```python
from build123d import *

# Parameters (mm, degrees)
SKETCH1_R           = 0.59563
SKETCH1_R_2         = 0.80645
BOSS_EXTRUDE1_DEPTH = 1.5
FILLET2_R           = 22
FILLET3_R           = 28
FILLET1_R           = 1


with BuildPart() as part:
    # Sketch1 → Boss-Extrude1 (new body)
    with BuildSketch(Plane.XY):
        Polygon((-2.5, -3.125), (-2.5, 3.875), (-2.5, 32.875), (27.5, 32.875), (27.5, 46.875), (32.5, 46.875), (32.5, 32.875), (32.5, 26.875), (2.5, 26.875), (2.5, 3.875), (2.5, -3.125), align=None)
        with Locations((0, 1.625)):
            Circle(SKETCH1_R, mode=Mode.SUBTRACT)
        with Locations((0, -1.625)):
            Circle(SKETCH1_R, mode=Mode.SUBTRACT)
        with Locations((30, 44.875)):
            Circle(SKETCH1_R_2, mode=Mode.SUBTRACT)
        with Locations((30, 34.875)):
            Circle(SKETCH1_R_2, mode=Mode.SUBTRACT)
    extrude(amount=BOSS_EXTRUDE1_DEPTH)

    # Fillet2
    fillet2_edges = [part.edges().sort_by_distance(p)[0] for p in [
        (2.5, 26.875, 0.75),
    ]]
    fillet(fillet2_edges, radius=FILLET2_R)

    # Fillet3
    fillet3_edges = [part.edges().sort_by_distance(p)[0] for p in [
        (-2.5, 32.875, 0.75),
    ]]
    fillet(fillet3_edges, radius=FILLET3_R)

    # Fillet1
    fillet1_edges = [part.edges().sort_by_distance(p)[0] for p in [
        (2.5, -3.125, 0.75),
        (-2.5, -3.125, 0.75),
        (27.5, 46.875, 0.75),
        (32.5, 46.875, 0.75),
        (32.5, 26.875, 0.75),
    ]]
    fillet(fillet1_edges, radius=FILLET1_R)


solid = part.part
```
Geometry: final body of the model. Coordinates: model frame, mm. A direction names the side the tool comes from. Coordinates: 2 decimals unless noted, no trailing zeros. Order: outer loops, then holes, each group sorted by start corner. A loop starts at its lowest first (then second) coordinate and runs counter-clockwise, first axis right, second up.
Item 1: Access query for faces 1 (the face through (30.434, 35.555, 0.74)), 2 (the face through (28, 26.875, 1)), 3 (the face through (27.5, 39, 1)). Directions: +Z, -Z, +X, -X, +Y, -Y. A direction counts if a zero-diameter tool reaches every point of the face in a straight line with its end or side. Return the directions, or none.
Answer:
face 1: +Z, -Z
face 2: +Z, -Z, +X, -Y
face 3: +Z, -Z, -X, +Y
Item 2: Contact query for flat-ended pins moving along their axis: P1, Ø1.4, axis at x = 0, y = -1.625, coming from the -Z side; P2, Ø0.8, axis at y = 38, z = 0.5, coming from the -X side; P3, Ø0.8, axis at x = 28.5, z = 1, coming from the -Y side (3 decimals); P4, Ø0.8, axis at y = 0, z = 1, coming from the +X side. Output: stop coordinate, or through.
Answer:
P1: stops at z = 0
P2: stops at x = 27.5
P3: stops at y = 26.875
P4: stops at x = 2.5
Item 3: Section query A-A (x = 30). Output: boundary loops of the cut face in (y, z) (3 decimals), then the cut area to 3 significant figures.
Answer:
outline: (26.875, 0) - (34.069, 0) - (34.069, 1.5) - (26.875, 1.5) - close; (35.681, 0) - (44.069, 0) - (44.069, 1.5) - (35.681, 1.5) - close; (45.681, 0) - (46.875, 0) - (46.875, 1.5) - (45.681, 1.5) - close
area: 25.2 mm2
Item 4: Draft query along Y for faces 4 (the face through (0, -3.125, 1)), 5 (the face through (30.434, 45.555, 0.74)), 6 (the face through (32.2, 46.59, 0.76)). Return one class per face: released by +Y, released by -Y, zero draft, split by the parting line, or undercut.
Answer:
face 4: released by -Y
face 5: undercut
face 6: released by +Y
Item 5: Section query C-C (y = 42). Output: boundary loops of the cut face in (x, z).
Answer:
outline: (27.5, 0) - (32.5, 0) - (32.5, 1.5) - (27.5, 1.5) - close
Item 6: Section query B-B (z = 0.95). Output: boundary loops of the cut face in (x, y) (3 decimals), then the cut area to 3 significant figures.
Answer:
outline: (-2.5, -2.125) arc R1 ccw to (-1.5, -3.125) - (1.5, -3.125) arc R1 ccw to (2.5, -2.125) - (2.5, 4.875) arc R22 cw to (24.5, 26.875) - (31.5, 26.875) arc R1 ccw to (32.5, 27.875) - (32.5, 45.875) arc R1 ccw to (31.5, 46.875) - (28.5, 46.875) arc R1 ccw to (27.5, 45.875) - (27.5, 32.875) - (25.5, 32.875) arc R28 ccw to (-2.5, 4.875) - close; hole circle Ø1.191 at (0, -1.625); hole circle Ø1.191 at (0, 1.625); hole circle Ø1.613 at (30, 34.875); hole circle Ø1.613 at (30, 44.875)
area: 358 mm2
Item 7: Section query D-D (x = 0). Output: boundary loops of the cut face in (y, z) (3 decimals).
Answer:
outline: (-3.125, 0) - (-2.221, 0) - (-2.221, 1.5) - (-3.125, 1.5) - close; (-1.029, 0) - (1.029, 0) - (1.029, 1.5) - (-1.029, 1.5) - close; (2.221, 0) - (16.44, 0) - (16.44, 1.5) - (2.221, 1.5) - close
Item 8: Material intervals for line 1 along Y through (x, z) = (30, 0.5) (3 decimals); line 2 along Y through (x, z) = (0, 0.95) (3 decimals); line 3 along Y through (x, z) = (28.5, 1.05) (3 decimals), sorted ascending.
Answer:
line 1: y = 26.875 to 34.069, 35.681 to 44.069, 45.681 to 46.875
line 2: y = -3.125 to -2.221, -1.029 to 1.029, 2.221 to 16.44
line 3: y = 26.875 to 46.875
